```python
from build123d import *

# Parameters (mm, degrees)
F0_R     = 9.525
F1_DEPTH = 19.05
F0_R_2   = 63.5
F2_DEPTH = 76.2
F0_R_3   = 31.75
F3_DEPTH = 19.05
F0_R_4   = 19.05
F4_DEPTH = 50.8
F0_R_5   = 6.35
F5_DEPTH = 38.1


with BuildPart() as f1:
    # F0 (on Top) → F1 (new body)
    with BuildSketch(Plane.XY):
        with BuildLine():
            ThreePointArc((0, -76.2), (-76.2, 0), (0, 76.2))
            Line((0, 76.2), (-107.95, 76.2))
            ThreePointArc((-107.95, 76.2), (-127, 57.15), (-107.95, 38.1))
            Line((-107.95, 38.1), (-88.9, 38.1))
            Line((-88.9, 38.1), (-88.9, -38.1))
            Line((-88.9, -38.1), (-107.95, -38.1))
            ThreePointArc((-107.95, -38.1), (-127, -57.15), (-107.95, -76.2))
            Line((-107.95, -76.2), (0, -76.2))
        make_face()
        with Locations((-107.95, -57.15)):
            Circle(F0_R, mode=Mode.SUBTRACT)
        with Locations((-107.95, 57.15)):
            Circle(F0_R, mode=Mode.SUBTRACT)
        with BuildLine():
            ThreePointArc((0, 76.2), (53.881537, 53.881537), (76.2, 0))
            ThreePointArc((76.2, 0), (53.881537, -53.881537), (0, -76.2))
            Line((0, -76.2), (107.95, -76.2))
            ThreePointArc((107.95, -76.2), (127, -57.15), (107.95, -38.1))
            Line((107.95, -38.1), (88.9, -38.1))
            Line((88.9, -38.1), (88.9, 38.1))
            Line((88.9, 38.1), (107.95, 38.1))
            ThreePointArc((107.95, 38.1), (127, 57.15), (107.95, 76.2))
            Line((107.95, 76.2), (0, 76.2))
        make_face()
        with Locations((107.95, -57.15)):
            Circle(F0_R, mode=Mode.SUBTRACT)
        with Locations((107.95, 57.15)):
            Circle(F0_R, mode=Mode.SUBTRACT)
    extrude(amount=F1_DEPTH)

    # F0 (on Top) → F2 (join)
    with BuildSketch(Plane.XY):
        with BuildLine():
            ThreePointArc((0, -76.2), (53.881537, -53.881537), (76.2, 0))
            ThreePointArc((76.2, 0), (53.881537, 53.881537), (0, 76.2))
            ThreePointArc((0, 76.2), (-76.2, 0), (0, -76.2))
        make_face()
        Circle(F0_R_2, mode=Mode.SUBTRACT)
    extrude(amount=F2_DEPTH)

    # F0 (on Top) → F3 (join)
    with BuildSketch(Plane.XY):
        Circle(F0_R_2)
        Circle(F0_R_3, mode=Mode.SUBTRACT)
    extrude(amount=F3_DEPTH)

    # F0 (on Top) → F4 (join)
    with BuildSketch(Plane.XY):
        Circle(F0_R_3)
        Circle(F0_R_4, mode=Mode.SUBTRACT)
    extrude(amount=F4_DEPTH)

    # F0 (on Top) → F5 (join)
    with BuildSketch(Plane.XY):
        Circle(F0_R_4)
        Circle(F0_R_5, mode=Mode.SUBTRACT)
    extrude(amount=F5_DEPTH)


solid = f1.part
```
Geometry: final body of the model. Coordinates: model frame, mm. A direction names the side the tool comes from. Coordinates: 2 decimals unless noted, no trailing zeros. Order: outer loops, then holes, each group sorted by start corner. A loop starts at its lowest first (then second) coordinate and runs counter-clockwise, first axis right, second up. Notation, with made-up numbers: (-25.75, 24) -> (-6.75, 24) arc R15 ccw to (-6.75, 42) -> close; hole circle Ø11 at (-3, 30). An arc over 180 degrees is marked (long way). Write each question's results on one line, items separated by ' | '. Start each with the question number.
1) Cut plane C-C, the plane x = -28. Output: boundary loops of the cut face in (y, z).
2) Mould query, pull axis X, two halves, no side actions, for faces 6 (the cylindrical face through (-126.995, 57.569, 9.392)), 7 (the flat face through (14, -14, 50.8)), 8 (the cylindrical face through (-114.97, -50.71, 9.39)), 9 (the flat face through (99, -38.1, 9)). Classes: released by +X, released by -X, zero draft, split by the parting line, or undercut.
3) Material intervals for line 1 along Y through (x, z) = (107.95, 7) (3 decimals); line 2 along X through (y, z) = (-57, 11); line 3 along Y through (x, z) = (-21, 30.5), sorted ascending.
4) Cut plane A-A, the plane z = 14.5. Output: boundary loops of the cut face in (x, y) (3 decimals).
5) Set-up query: faces 1 (the flat face through (2, 76.2, 9)), 2 (the flat face through (82, 0, 19.05)), 3 (the flat face through (-98, -38.1, 9)), 4 (the flat face through (-5, 5, 38.1)), 5 (the flat face through (-78, 0, 19.05)). Return all of +Z, -Z, +X, -X, +Y, -Y with unobstructed straight access to the full face (end or side cutting, diameter ignored); none if empty.
6) Cut plane B-B, the plane y = 57.15. Output: boundary loops of the cut face in (x, z) (3 decimals), and give its area (3 significant figures).
7) First-contact query: pin 1 (2 mm diameter, centred on x = -17, y = -54, fed in from +Z); pin 2 (12 mm diameter, centred on y = 37.5, z = 40, fed in from +X); pin 3 (10 mm diameter, centred on y = -8, z = 32, fed in from -X); pin 4 (15 mm diameter, centred on x = 107.95, y = 57.15, fed in from -Z). Flat tips, straight axial feed; report the tip coordinate or a pass-through.
8) Cut plane D-D, the plane z = 71. Output: boundary loops of the cut face in (x, y), and give its area (3 significant figures).
Checks:
1) outline: (-76.2, 0) -> (76.2, 0) -> (76.2, 19.05) -> (70.87, 19.05) -> (70.87, 76.2) -> (56.99, 76.2) -> (56.99, 19.05) -> (14.97, 19.05) -> (14.97, 50.8) -> (-14.97, 50.8) -> (-14.97, 19.05) -> (-56.99, 19.05) -> (-56.99, 76.2) -> (-70.87, 76.2) -> (-70.87, 19.05) -> (-76.2, 19.05) -> close
2) face 6: released by -X | face 7: undercut | face 8: undercut | face 9: zero draft
3) line 1: -76.2 to -66.675, -47.625 to -38.1, 38.1 to 47.625, 66.675 to 76.2 | line 2: -127 to -117.47, -98.43 to 98.43, 117.47 to 127 | line 3: -73.25 to -59.93, -23.81 to 23.81, 59.93 to 73.25
4) outline: (-107.95, -76.2) -> (107.95, -76.2) arc R19.05 ccw to (107.95, -38.1) -> (88.9, -38.1) -> (88.9, 38.1) -> (107.95, 38.1) arc R19.05 ccw to (107.95, 76.2) -> (-107.95, 76.2) arc R19.05 ccw to (-107.95, 38.1) -> (-88.9, 38.1) -> (-88.9, -38.1) -> (-107.95, -38.1) arc R19.05 ccw to start; hole circle Ø19.05 at (-107.95, -57.15); hole circle Ø19.05 at (-107.95, 57.15); hole circle Ø12.7 at (0, 0); hole circle Ø19.05 at (107.95, -57.15); hole circle Ø19.05 at (107.95, 57.15)
5) face 1: +Z, -Z, +X, -X, +Y | face 2: +Z, +X | face 3: +Z, -Z, -X | face 4: +Z | face 5: +Z, -X
6) outline: (-127, 0) -> (-117.475, 0) -> (-117.475, 19.05) -> (-127, 19.05) -> close; (-98.425, 0) -> (98.425, 0) -> (98.425, 19.05) -> (50.402, 19.05) -> (50.402, 76.2) -> (27.679, 76.2) -> (27.679, 19.05) -> (-27.679, 19.05) -> (-27.679, 76.2) -> (-50.402, 76.2) -> (-50.402, 19.05) -> (-98.425, 19.05) -> close; (117.475, 0) -> (127, 0) -> (127, 19.05) -> (117.475, 19.05) -> close | area: 6,710 mm^2
7) pin 1: z = 19.05 | pin 2: x = 69.38 | pin 3: x = -76.14 | pin 4: through
8) outline: (0, -76.2) arc R76.2 ccw to (76.2, 0) arc R76.2 ccw (long way) to start; hole circle Ø127 at (0, 0) | area: 5,570 mm^2
